Input: dimensioned drawing with shaded views. Units: mm. Origin: part minimum x, y, z. A direction names the side the tool comes from. Coordinates: 2 decimals unless noted, no trailing zeros. Order: outer loops, then holes, each group sorted by start corner. A loop starts at its lowest first (then second) coordinate and runs counter-clockwise, first axis right, second up. Notation, with made-up numbers: (-14, 27.5) - (28, 27.5) arc R9 ccw to (28, 35.5) - close; hole circle Ø11 at (47, 52). An arc over 180 degrees is marked (long way). One line per question, with ' | ' between items. Start each with the question number.
(1) Section A-A (x = 12.9). Return the cut outline in (y, z).
(2) Draft query along Y for the marked faces 1, 2 and 3. Return one class per face: +Y half, -Y half, draft (parallel to the pull), parting line (faces both ways), or undercut.
(3) Access query for the marked faces 4, 5 and 6. Directions: +Z, -Z, +X, -X, +Y, -Y. A direction counts if a zero-diameter tool reaches every point of the face in a straight line with its end or side. Return the directions, or none.
(4) Contact query for flat-ended pins moving along their axis: P1, Ø1, axis at y = 7.5, z = 9.5, coming from the -X side; P2, Ø1.5, axis at x = 12.5, z = 11.5, coming from the +Y side; P3, Ø1, axis at y = 14, z = 9, coming from the +X side. Output: stop coordinate, or through.
(5) Section B-B (y = 12.9). Return the cut outline in (x, z).
(6) Line query: line 1 along Z through (x, y) = (4.25, 3.5); line 2 along Z through (x, y) = (12.9, 18.5); line 3 along Z through (x, y) = (22.5, 11.5). Output: solid intervals per line, ascending.
(7) Section C-C (y = 17.5). Return the cut outline in (x, z), then the cut area to 3 significant figures.
(8) Section D-D (x = 23). Return the cut outline in (y, z).
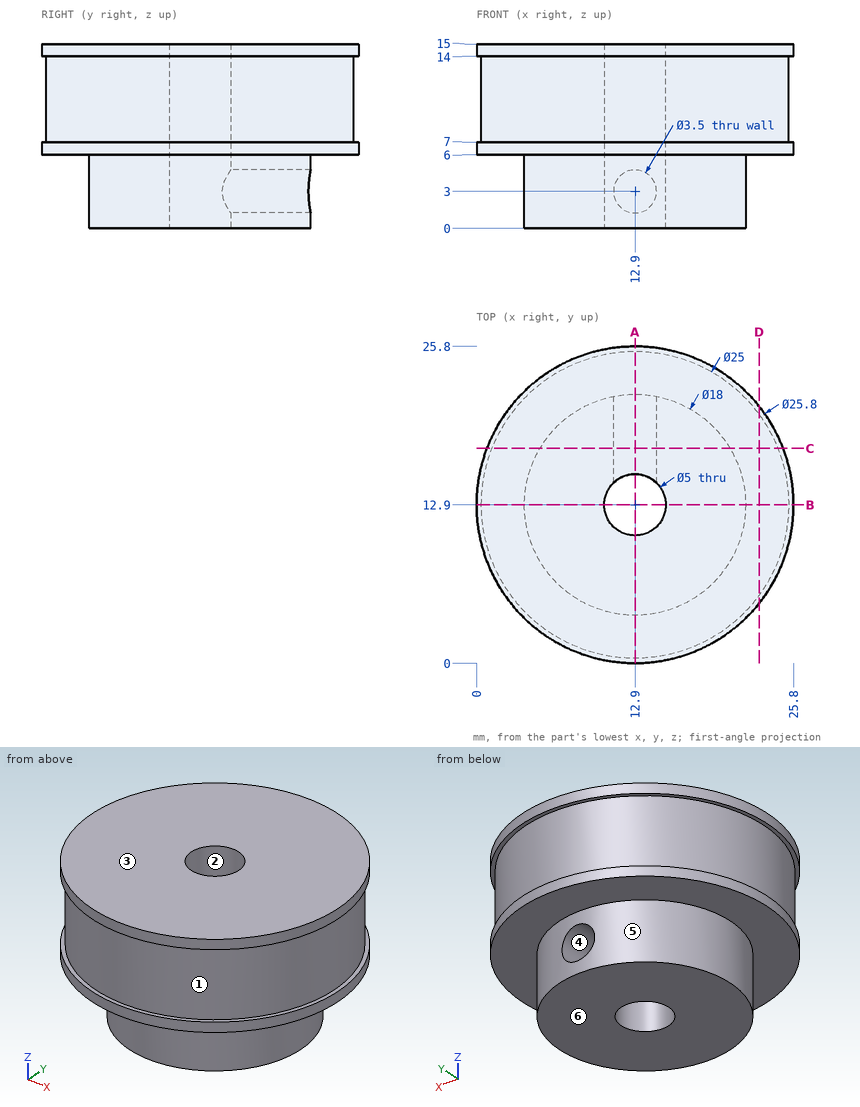
Response values:
1) outline: (0, 6) - (3.9, 6) - (3.9, 0) - (10.4, 0) - (10.4, 15) - (0, 15) - (0, 14) - (0.4, 14) - (0.4, 7) - (0, 7) - close; (15.4, 0) - (21.9, 0) - (21.9, 1.25) - (15.4, 1.25) - close; (15.4, 4.75) - (21.9, 4.75) - (21.9, 6) - (25.8, 6) - (25.8, 7) - (25.4, 7) - (25.4, 14) - (25.8, 14) - (25.8, 15) - (15.4, 15) - close
2) face 1: parting line | face 2: undercut | face 3: draft
3) face 4: +Y | face 5: -Z | face 6: -Z, +X, -X, +Y, -Y
4) P1: stops at x = 1.4 | P2: stops at y = 25.4 | P3: stops at x = 25.39
5) outline: (0, 6) - (3.9, 6) - (3.9, 0) - (10.4, 0) - (10.4, 15) - (0, 15) - (0, 14) - (0.4, 14) - (0.4, 7) - (0, 7) - close; (15.4, 0) - (21.9, 0) - (21.9, 6) - (25.8, 6) - (25.8, 7) - (25.4, 7) - (25.4, 14) - (25.8, 14) - (25.8, 15) - (15.4, 15) - close
6) line 1: z = 6 to 7, 14 to 15 | line 2: z = 0 to 1.25, 4.75 to 15 | line 3: z = 6 to 15
7) outline: (0.85, 6) - (5.16, 6) - (5.16, 0) - (20.64, 0) - (20.64, 6) - (24.95, 6) - (24.95, 7) - (24.52, 7) - (24.52, 14) - (24.95, 14) - (24.95, 15) - (0.85, 15) - (0.85, 14) - (1.28, 14) - (1.28, 7) - (0.85, 7) - close; hole circle Ø3.5 at (12.9, 3) | area: 294 mm²
8) outline: (4.88, 6) - (20.92, 6) - (20.92, 7) - (20.26, 7) - (20.26, 14) - (20.92, 14) - (20.92, 15) - (4.88, 15) - (4.88, 14) - (5.54, 14) - (5.54, 7) - (4.88, 7) - close
